```python
from build123d import *

# Parameters (mm, degrees)
SKETCH1_R           = 1.65
SKETCH1_R_2         = 1.6
BOSS_EXTRUDE1_DEPTH = 3


with BuildPart() as part:
    # Sketch1 → Boss-Extrude1 (new body)
    with BuildSketch(Plane.XY):
        with BuildLine():
            Line((22.650283011, 50.925569007), (22.650283011, 36.440298517))
            ThreePointArc((22.650283011, 36.440298517), (30.012998862, 32.222429945), (34.230867434, 39.585145796))
            Line((34.230867434, 39.585145796), (34.230867434, 89.585145796))
            Line((34.230867434, 89.585145796), (27.230867434, 98.07042717))
            Line((27.230867434, 98.07042717), (19.230867434, 98.07042717))
            Line((19.230867434, 98.07042717), (19.230867434, 55.070526621))
            Line((19.230867434, 55.070526621), (22.650283011, 50.925569007))
        make_face()
        with Locations((28.440575223, 38.012722157)):
            Circle(SKETCH1_R, mode=Mode.SUBTRACT)
        with Locations((26.230867434, 89.07042717)):
            Circle(SKETCH1_R_2, mode=Mode.SUBTRACT)
    extrude(amount=BOSS_EXTRUDE1_DEPTH)


solid = part.part
```
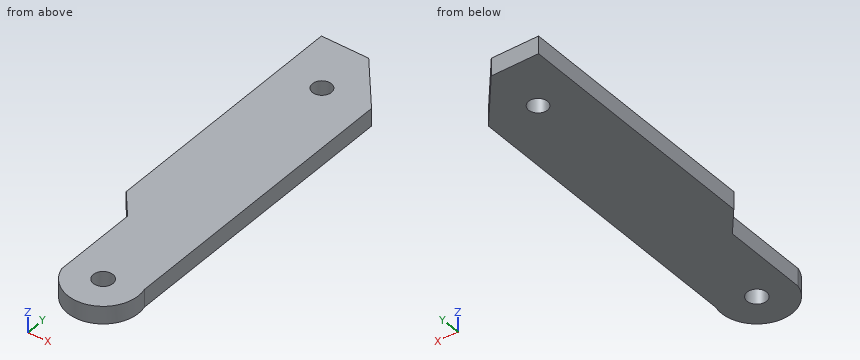
Geometry check sheet. Reference: the model listing, model coordinates, mm. Give positions to 0.01 mm unless a question says otherwise; leave off trailing zeros. Loops run counter-clockwise (first coordinate to the right, second up) from the corner with the lowest first, then second, coordinate; pieces in that order, holes last. Notation, with made-up numbers: (47, 44) - (85, 44) arc R16 cw to (85, 75) - close; hole circle Ø11 at (55, -25). An arc over 180 degrees is marked (long way). Use CSV: the item, a comma, the result in double quotes. Start each with the question number.
Q1. Section check D-D, the plane y = 54. Record the cut outline in (x, z).
Q2. Go/stop test with flat-tipped pins: pin 1 Ø3 at (x, y) = (28.44, 38.01) entering from -Z; pin 2 Ø0.9 at (y, z) = (46, 1.5) entering from -X. Record where each tip stops, or that it passes through.
Q3. Section check A-A, the plane x = 29.5. Record the cut outline in (y, z), and give its area (3 significant figures).
Q4. Section check C-C, the plane y = 42.5. Record the cut outline in (x, z), and give its area (3 significant figures).
Q5. Scan lines: probe 1 along Y at (x, z) = (27.5, 0.35); probe 2 along X at (y, z) = (83.5, 0.45); probe 3 along X at (y, z) = (49, 0.4). Record each from-to range of solid material in increasing order. Write a range as from..to.
Q6. Section check B-B, the plane z = 2.1. Record the cut outline in (x, y), and give its area (3 significant figures).
Findings below:
1,outline,"(20.11, 0) - (34.23, 0) - (34.23, 3) - (20.11, 3) - close"
2,pin 1,"passes through"
2,pin 2,"stops at x = 22.65"
3,outline,"(32.11, 0) - (36.75, 0) - (36.75, 3) - (32.11, 3) - close; (39.28, 0) - (95.32, 0) - (95.32, 3) - (39.28, 3) - close"
3,area,"182 mm^2"
4,outline,"(22.65, 0) - (34.23, 0) - (34.23, 3) - (22.65, 3) - close"
4,area,"34.7 mm^2"
5,probe 1,"y = 32.09..36.66, 39.37..88.1, 90.04..97.74"
5,probe 2,"x = 19.23..34.23"
5,probe 3,"x = 22.65..34.23"
6,outline,"(19.23, 55.07) - (22.65, 50.93) - (22.65, 36.44) arc R6 ccw to (34.23, 39.59) - (34.23, 89.59) - (27.23, 98.07) - (19.23, 98.07) - close; hole circle Ø3.2 at (26.23, 89.07); hole circle Ø3.3 at (28.44, 38.01)"
6,area,"860 mm^2"
